Model file for the job. Use its own axes, mm. Round coordinates to 2 decimals unless told otherwise and drop trailing zeros. Order: outer loops, then holes, each group sorted by start corner. A loop starts at its lowest first (then second) coordinate and runs counter-clockwise, first axis right, second up. Notation, with made-up numbers: (68.5, -0.5) - (91.5, -0.5) arc R10 ccw to (91.5, 3.5) - close; hole circle Ø5 at (38.25, 12). An arc over 180 degrees is marked (long way). Put each result on its own line as item: value. Start each with the question number.
Item 1: Probe probe 1 along X at (y, z) = (1.95, -66.2) (3 decimals); probe 2 along X at (y, z) = (1.6, 0) (3 decimals); probe 3 along X at (y, z) = (0.75, 0.5). List the from-to ranges inside material, lowest first.
Item 2: Saw through at C-C on z = 44. List the corners of the cut face in (x, y) (3 decimals).
Item 3: Pin check, flat tip, straight feed: pin 1 Ø4.5 at (x, z) = (0, -63.5) entering from +Y. Stop position of the tip, or through.
Item 4: Saw through at B-B on y = 0.7. State how many separate pieces and enclosed holes the cut face has, plus the area to 3 significant figures.
Item 5: Saw through at A-A on x = 14. List the corners of the cut face in (y, z) (3 decimals).
```python
from build123d import *

# Parameters (mm, degrees)
SKETCH2_W           = 152.4
SKETCH2_H           = 152.4
SKETCH2_R           = 50.8
BOSS_EXTRUDE1_DEPTH = 3.175
CUT_EXTRUDE1_REACH  = 109.81
SKETCH3_R           = 2.665000004
CUT_EXTRUDE2_REACH  = 109.81
SKETCH4_R           = 2.665000004


with BuildPart() as part:
    # Sketch2 → Boss-Extrude1 (new body)
    with BuildSketch(Plane(origin=(0, 0, 0), x_dir=(1, 0, 0), z_dir=(0, 1, 0))):
        Rectangle(SKETCH2_W, SKETCH2_H)
        with Locations(Location((0, 0, 0), (0, 0, 270))):
            Circle(SKETCH2_R, mode=Mode.SUBTRACT)
    extrude(amount=BOSS_EXTRUDE1_DEPTH)

    # Sketch3 → Cut-Extrude1 (cut, up to next)
    with BuildSketch(Plane(origin=(0, 3.175, 0), x_dir=(1, 0, 0), z_dir=(0, 1, 0)), mode=Mode.PRIVATE) as cut_extrude1_sk1:
        with Locations(Location((-66.2, -66.2, 0), (0, 0, 270))):
            Circle(SKETCH3_R)
    cut_extrude1_tool1 = extrude(cut_extrude1_sk1.sketch, amount=-CUT_EXTRUDE1_REACH, mode=Mode.PRIVATE) & part.part
    # Sketch3 → Cut-Extrude1 (cut, up to next)
    with BuildSketch(Plane(origin=(0, 3.175, 0), x_dir=(1, 0, 0), z_dir=(0, 1, 0)), mode=Mode.PRIVATE) as cut_extrude1_sk2:
        with Locations(Location((-66.2, 66.2, 0), (0, 0, 90))):
            Circle(SKETCH3_R)
    cut_extrude1_tool2 = extrude(cut_extrude1_sk2.sketch, amount=-CUT_EXTRUDE1_REACH, mode=Mode.PRIVATE) & part.part
    # Sketch3 → Cut-Extrude1 (cut, up to next)
    with BuildSketch(Plane(origin=(0, 3.175, 0), x_dir=(1, 0, 0), z_dir=(0, 1, 0)), mode=Mode.PRIVATE) as cut_extrude1_sk3:
        with Locations(Location((66.2, 66.2, 0), (0, 0, 270))):
            Circle(SKETCH3_R)
    cut_extrude1_tool3 = extrude(cut_extrude1_sk3.sketch, amount=-CUT_EXTRUDE1_REACH, mode=Mode.PRIVATE) & part.part
    # Sketch3 → Cut-Extrude1 (cut, up to next)
    with BuildSketch(Plane(origin=(0, 3.175, 0), x_dir=(1, 0, 0), z_dir=(0, 1, 0)), mode=Mode.PRIVATE) as cut_extrude1_sk4:
        with Locations(Location((66.2, -66.2, 0), (0, 0, 90))):
            Circle(SKETCH3_R)
    cut_extrude1_tool4 = extrude(cut_extrude1_sk4.sketch, amount=-CUT_EXTRUDE1_REACH, mode=Mode.PRIVATE) & part.part
    add(cut_extrude1_tool1.solids().sort_by_distance((-66.2, 3.175, 66.2))[0], mode=Mode.SUBTRACT)
    add(cut_extrude1_tool2.solids().sort_by_distance((-66.2, 3.175, -66.2))[0], mode=Mode.SUBTRACT)
    add(cut_extrude1_tool3.solids().sort_by_distance((66.2, 3.175, -66.2))[0], mode=Mode.SUBTRACT)
    add(cut_extrude1_tool4.solids().sort_by_distance((66.2, 3.175, 66.2))[0], mode=Mode.SUBTRACT)

    # Sketch4 → Cut-Extrude2 (cut, up to next)
    with BuildSketch(Plane(origin=(0, 3.175, 0), x_dir=(1, 0, 0), z_dir=(0, 1, 0)), mode=Mode.PRIVATE) as cut_extrude2_sk1:
        with Locations(Location((0, 63.5, 0), (0, 0, 270))):
            Circle(SKETCH4_R)
    cut_extrude2_tool1 = extrude(cut_extrude2_sk1.sketch, amount=-CUT_EXTRUDE2_REACH, mode=Mode.PRIVATE) & part.part
    # Sketch4 → Cut-Extrude2 (cut, up to next)
    with BuildSketch(Plane(origin=(0, 3.175, 0), x_dir=(1, 0, 0), z_dir=(0, 1, 0)), mode=Mode.PRIVATE) as cut_extrude2_sk2:
        with Locations(Location((-63.5, 0, 0), (0, 0, 270))):
            Circle(SKETCH4_R)
    cut_extrude2_tool2 = extrude(cut_extrude2_sk2.sketch, amount=-CUT_EXTRUDE2_REACH, mode=Mode.PRIVATE) & part.part
    # Sketch4 → Cut-Extrude2 (cut, up to next)
    with BuildSketch(Plane(origin=(0, 3.175, 0), x_dir=(1, 0, 0), z_dir=(0, 1, 0)), mode=Mode.PRIVATE) as cut_extrude2_sk3:
        with Locations(Location((0, -63.5, 0), (0, 0, 270))):
            Circle(SKETCH4_R)
    cut_extrude2_tool3 = extrude(cut_extrude2_sk3.sketch, amount=-CUT_EXTRUDE2_REACH, mode=Mode.PRIVATE) & part.part
    # Sketch4 → Cut-Extrude2 (cut, up to next)
    with BuildSketch(Plane(origin=(0, 3.175, 0), x_dir=(1, 0, 0), z_dir=(0, 1, 0)), mode=Mode.PRIVATE) as cut_extrude2_sk4:
        with Locations(Location((63.5, 0, 0), (0, 0, 270))):
            Circle(SKETCH4_R)
    cut_extrude2_tool4 = extrude(cut_extrude2_sk4.sketch, amount=-CUT_EXTRUDE2_REACH, mode=Mode.PRIVATE) & part.part
    add(cut_extrude2_tool1.solids().sort_by_distance((0, 3.175, -63.5))[0], mode=Mode.SUBTRACT)
    add(cut_extrude2_tool2.solids().sort_by_distance((-63.5, 3.175, 0))[0], mode=Mode.SUBTRACT)
    add(cut_extrude2_tool3.solids().sort_by_distance((0, 3.175, 63.5))[0], mode=Mode.SUBTRACT)
    add(cut_extrude2_tool4.solids().sort_by_distance((63.5, 3.175, 0))[0], mode=Mode.SUBTRACT)


solid = part.part
```
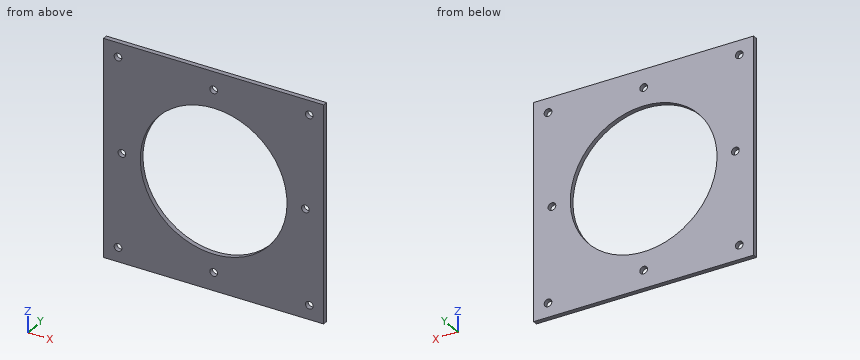
Results found:
1. probe 1: x = -76.2 to -68.865, -63.535 to 63.535, 68.865 to 76.2
1. probe 2: x = -76.2 to -66.165, -60.835 to -50.8, 50.8 to 60.835, 66.165 to 76.2
1. probe 3: x = -76.2 to -66.12, -60.88 to -50.8, 50.8 to 60.88, 66.12 to 76.2
2. outline: (-76.2, 0) - (-25.39, 0) - (-25.39, 3.175) - (-76.2, 3.175) - close; (25.39, 0) - (76.2, 0) - (76.2, 3.175) - (25.39, 3.175) - close
3. pin 1: passes through
4. separate pieces: 1
4. enclosed holes: 9
4. area: 14,900 mm²
5. outline: (0, -76.2) - (3.175, -76.2) - (3.175, -48.833) - (0, -48.833) - close; (0, 48.833) - (3.175, 48.833) - (3.175, 76.2) - (0, 76.2) - close
